Autodesk Inventor part; units mm, degrees
ref_plane "YZ Plane" through (0, 0, 0) normal (1, 0, 0) x (0, 1, 0)
ref_plane "XZ Plane" through (0, 0, 0) normal (0, 1, 0) x (-1, 0, 0)
ref_plane "XY Plane" through (0, 0, 0) normal (0, 0, 1) x (1, 0, 0)
sketch "Sketch1" plane through (0, 0, 0) normal (0, 0, 1) x (1, 0, 0)
  line L0 (0, 0) -> (-160, 0)
  line L1 (-160, 0) -> (-160, 300)
  line L2 (-160, 300) -> (0, 300)
  line L3 (0, 300) -> (0, 0)
  dimension "d0" = 160
  dimension "d1" = 300
extrude "Extrusion1" add sketch "Sketch1" along normal blind 10
sketch "Sketch2" plane through (0, 0, 10) normal (0, 0, 1) x (1, 0, 0)
  circle A0 centre (-130, 15) radius 2.55
  line L0 (-160, 0) -> (0, 0)
  line L1 (-160, 300) -> (-160, 0)
  circle A1 centre (-44, 15) radius 2.55
  circle A2 centre (-130, 149) radius 2.55
  circle A3 centre (-44, 149) radius 2.55
  circle A4 centre (-80, 250) radius 4.5984
  circle A5 centre (-50, 50) radius 5.0648 construction
  line L2 (0, 300) -> (-160, 300)
  line L3 (0, 0) -> (0, 300)
  dimension "d4" = 15
  dimension "d5" = 5.1
  dimension "d6" = 30
  dimension "d9" = 86
  dimension "d12" = 134
  dimension "d18" = 50
  dimension "d19" = 50
  dimension "d20" = 50
  dimension "d33" = 80
extrude "Extrusion2" cut sketch "Sketch2" against normal through all contours A0 | A1 | A2 | A3 | A4
chamfer "Chamfer1" distance 40 angle 45 3 edges at (0, 0, 5) (-160, 300, 5) (0, 300, 5)
sketch "Sketch3" plane through (0, 0, 0) normal (0, 0, -1) x (-1, 0, 0)
  line L0 (0, 300) -> (120, 300)
  line L1 (160, 260) -> (160, 0)
  line L2 (0, 0) -> (160, 300) construction
  circle A0 centre (94.1176, 176.4706) radius 2
  circle A1 centre (23.5294, 44.1176) radius 2
  line L3 (160, 0) -> (40, 0)
  line L4 (160, 0) -> (0, 0) construction
  line L5 (0, 260) -> (0, 0) construction
  line L6 (40, 300) -> (160, 300)
  line L7 (160, 300) -> (160, 0)
  dimension "d25" = 4
  dimension "d27" = 4
  dimension "d31" = 150
  dimension "d32" = 50
extrude "Extrusion3" cut sketch "Sketch3" against normal blind 10
properties part number "legno" material "Wood (Birch)"
The listing builds one solid part. Answer for the finished solid, in the listing's coordinates (mm). Coordinates: 2 decimals unless noted, no trailing zeros. Loops run counter-clockwise (first coordinate to the right, second up) from the corner with the lowest first, then second, coordinate; pieces in that order, holes last. Notation, with made-up numbers: (39, 54) -> (75, 54) arc R31 ccw to (75, 86) -> close; hole circle Ø10 at (51, -4.75). An arc over 180 degrees is marked (long way). Write item = value, one per line. Start each with the question number.
1) A cutting plane is placed at D-D (x = -29). Give the vertices of the cut face in (y, z).
2) A cutting plane is placed at B-B (x = -80). Give the vertices of the cut face in (y, z).
3) A cutting plane is placed at A-A (y = 250). Give the vertices of the cut face in (x, z), then the cut area to 3 significant figures.
4) Given pin 1 Ø2 at (x, z) = (-135, 5) entering from +Y; pin 2 Ø2 at (x, z) = (-131.5, 6.5) entering from +Y, each flat-ended and moving along its own axis, determine where each tip first touches the part or whether it passes through.
5) The mould has two halves that part along X. Classify faces 1 (the face through (-83.389, 253.108, 5.07)), 2 (the face through (-20, 20, 5)), 3 (the face through (-81, 152, 10)): released by +X, released by -X, zero draft, split by the parting line, or undercut.
6) Straight lines are drawn through the part: line 1 (X direction, y = 149, z = 3); line 2 (Y direction, x = -44, z = 4.75); line 3 (Y direction, x = -80, z = 2.25). For each, find the intervals that lie inside material, in ascending order. Write a range as from..to.
7) A cutting plane is placed at C-C (z = 2.5). Give the vertices of the cut face in (x, y).
Responses:
q1.outline = (11, 0) -> (289, 0) -> (289, 10) -> (11, 10) -> close
q2.outline = (0, 0) -> (245.4, 0) -> (245.4, 10) -> (0, 10) -> close; (254.6, 0) -> (300, 0) -> (300, 10) -> (254.6, 10) -> close
q3.outline = (-160, 0) -> (-84.6, 0) -> (-84.6, 10) -> (-160, 10) -> close; (-75.4, 0) -> (0, 0) -> (0, 10) -> (-75.4, 10) -> close
q3.area = 1,510 mm²
q4.pin_1 = 286
q4.pin_2 = 289.5
q5.face_1 = undercut
q5.face_2 = released by +X
q5.face_3 = zero draft
q6.line_1 = -160..-132.55, -127.45..-46.55, -41.45..0
q6.line_2 = 0..12.45, 17.55..146.45, 151.55..300
q6.line_3 = 0..245.4, 254.6..300
q7.outline = (-160, 0) -> (-40, 0) -> (0, 40) -> (0, 260) -> (-40, 300) -> (-120, 300) -> (-160, 260) -> close; hole circle Ø5.1 at (-130, 15); hole circle Ø5.1 at (-130, 149); hole circle Ø4 at (-94.12, 176.47); hole circle Ø9.2 at (-80, 250); hole circle Ø5.1 at (-44, 15); hole circle Ø5.1 at (-44, 149); hole circle Ø4 at (-23.53, 44.12)
